Could you check a few things on this drawing? It's one solid part, dimensions in mm from its lowest x, y, z. Coordinates: 2 decimals unless noted, no trailing zeros. Order: outer loops, then holes, each group sorted by start corner. A loop starts at its lowest first (then second) coordinate and runs counter-clockwise, first axis right, second up.
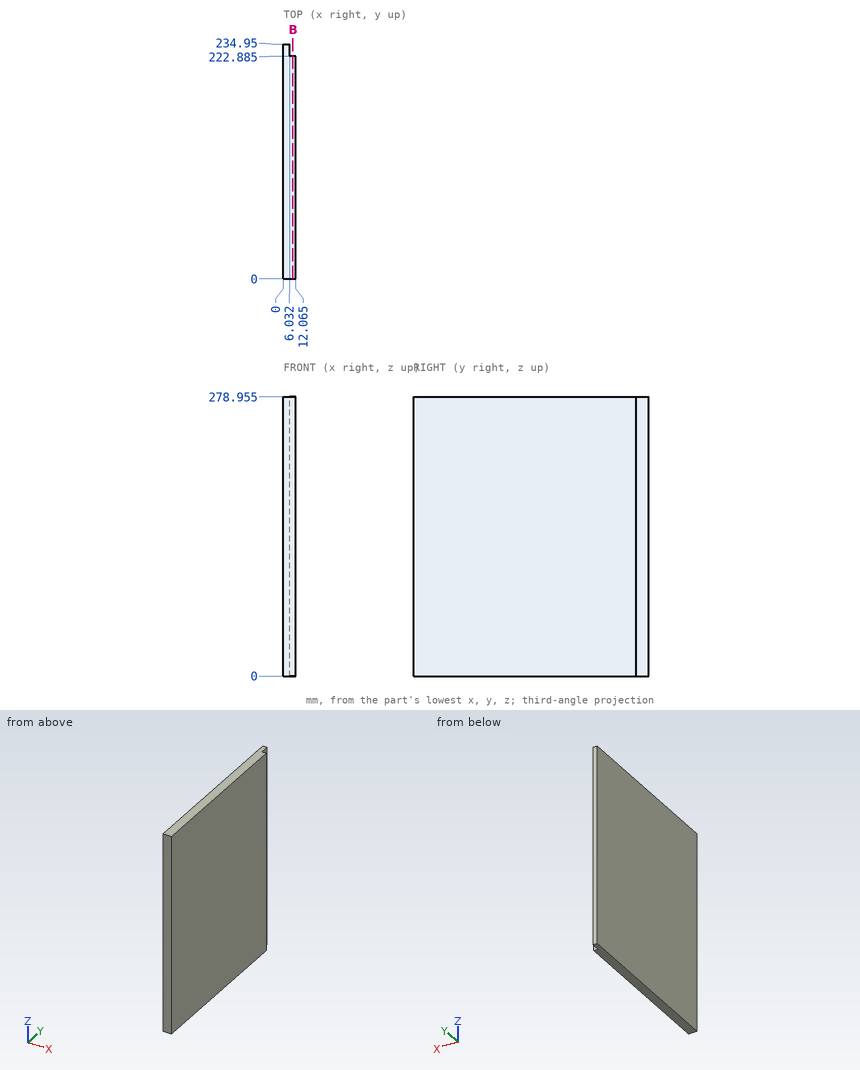
Q1. I need wall thicknesses on L1, parallel to Y at x = 7, z = 79.5 (1 decimal). Which ranges of the line are inside material? Lowest first, please.
Q2. If we section it at B-B on x = 9.5: Write out the boundary of the cut face in (y, z) (1 decimal), then the cut area to 3 significant figures.
Q3. Will these pins go through, and if not, where does the flat tip stop? pin 1 (6.5 mm diameter, centred on x = 9.5, z = 196.5, fed in from +Y) (1 decimal); pin 2 (6 mm diameter, centred on y = 226, z = 141.5, fed in from +X).
Reply:
1. L1: y = 0 to 222.9
2. outline: (0, 0) - (222.9, 0) - (222.9, 279) - (0, 279) - close
2. area: 62,200 mm2
3. pin 1: stops at y = 222.9
3. pin 2: stops at x = 6.03
